For this review, take the finished solid that the model builds, in its own axes (mm). Face numbers are marked on the shaded views. A direction names the side the tool comes from. Coordinates: 2 decimals unless noted, no trailing zeros. Write each loop counter-clockwise with the first axis right and the second up, starting at its lowest first coordinate (ties: lowest second). Pieces come first, ordered by that corner, then holes. Notation, with made-up numbers: M 74.25,3.5 L 126.25,3.5 A20 cw 126.25,33.5 Z; hole C -1,31 d5. An arc over 180 degrees is marked long. One line per question, with ' | ' between items.
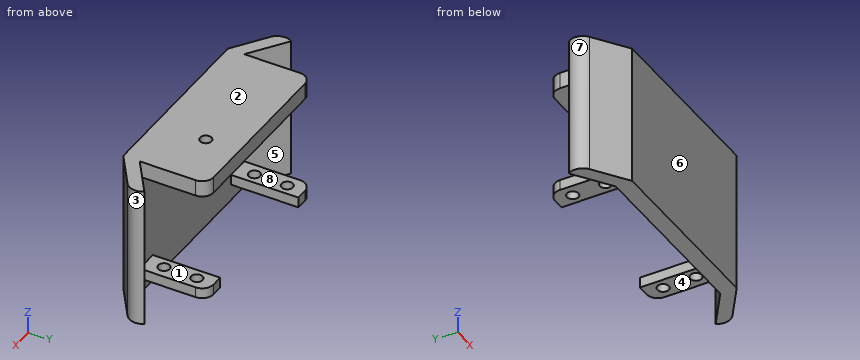
from build123d import *

# Parameters (mm, degrees)
SKETCH1_W            = 55.5
SKETCH1_H            = 43.2
BASE_DEPTH           = 5
SKETCH2_W            = 55.5
SKETCH2_H            = 25.5
WALL_DEPTH           = 5
SKETCH3_W            = 7
SKETCH3_H            = 20.5
MOUNTINGTABS_DEPTH   = 5
LIPS_REACH           = 76.811
SKETCH5_R            = 1.75
MOUNTINGHOLES_DEPTH  = 5
FILLETS_R            = 3.5
SKETCH6_R            = 1.75
THROUGHHOLE_DEPTH    = 5
MIRROR1_START        = -40
MIRROR1_OUTLINE_R    = 1.75
MIRROR1_DEPTH        = 1.8
MIRROR1_START_2      = -38.2
MIRROR1_2_OUTLINE_R  = 1.75
MIRROR1_2_DEPTH      = 3.2
FILLETS_OF_MIRROR2_R = 3.5
CUT_EXTRUDE2_DEPTH   = 5
CUT_EXTRUDE3_DEPTH   = 3.2


# Read off the part's stored shape, not the designer's step: Mirror1
with BuildPart() as part:
    # Sketch1 → base (new body)
    with BuildSketch(Plane(origin=(0, 0, 0), x_dir=(1, 0, 0), z_dir=(0, 1, 0))):
        with Locations((27.75, 21.6)):
            Rectangle(SKETCH1_W, SKETCH1_H)
    extrude(amount=BASE_DEPTH)

    # Sketch2 → wall (add)
    with BuildSketch(Plane(origin=(0, 0, -43.2), x_dir=(-1, 0, 0), z_dir=(0, 0, -1))):
        with Locations((-27.75, 12.75)):
            Rectangle(SKETCH2_W, SKETCH2_H)
    wall = extrude(amount=-WALL_DEPTH)

    # Sketch3 → mountingTabs (add)
    with BuildSketch(Plane.XY.offset(-8.2)):
        with Locations((3.5, 15.25)):
            Rectangle(SKETCH3_W, SKETCH3_H)
        with Locations((52, 15.25)):
            Rectangle(SKETCH3_W, SKETCH3_H)
    extrude(amount=MOUNTINGTABS_DEPTH)

    # lips: up to this face of the body (flat: up to its plane)
    lips_end = Plane(part.part.faces().sort_by_distance((27.75, 12.75, -43.2))[0])
    # Sketch4 → lips (add, up to the picked face)
    with BuildSketch(Plane.XY, mode=Mode.PRIVATE) as lips_sk1:
        with BuildLine():
            Line((0, 0), (-10.208884478, 7.148337868))
            ThreePointArc((-10.208884478, 7.148337868), (-11.894564223, 9.792816133), (-11.218174515, 12.85505036))
            Line((-11.218174515, 12.85505036), (0, 5))
            Line((0, 5), (0, 0))
        make_face()
    lips_tool1 = split(extrude(lips_sk1.sketch, amount=-LIPS_REACH, mode=Mode.PRIVATE), bisect_by=lips_end, keep=Keep.BOTH, mode=Mode.PRIVATE)
    # Sketch4 → lips (add, up to the picked face)
    with BuildSketch(Plane.XY, mode=Mode.PRIVATE) as lips_sk2:
        with BuildLine():
            Line((55.5, 5), (66.718174515, 12.85505036))
            ThreePointArc((66.718174515, 12.85505036), (67.394564223, 9.792816133), (65.708884478, 7.148337868))
            Line((65.708884478, 7.148337868), (55.5, 0))
            Line((55.5, 0), (55.5, 5))
        make_face()
    lips_tool2 = split(extrude(lips_sk2.sketch, amount=-LIPS_REACH, mode=Mode.PRIVATE), bisect_by=lips_end, keep=Keep.BOTH, mode=Mode.PRIVATE)
    add(lips_tool1.solids().sort_by(Axis((-5.839287, 6.590277, 0), (0, 0, -1)))[0])
    add(lips_tool2.solids().sort_by(Axis((61.339287, 6.590277, 0), (0, 0, -1)))[0])

    # Sketch5 → mountingHoles (cut)
    with BuildSketch(Plane.XY.offset(-3.2)):
        with Locations((3.75, 20.25)):
            Circle(SKETCH5_R)
        with Locations(Location((3.75, 10.25, 0), (0, 0, 180))):
            Circle(SKETCH5_R)
        with Locations((51.75, 10.25)):
            Circle(SKETCH5_R)
        with Locations(Location((51.75, 20.25, 0), (0, 0, 180))):
            Circle(SKETCH5_R)
    extrude(amount=-MOUNTINGHOLES_DEPTH, mode=Mode.SUBTRACT)

    # fillets
    fillets_edges = [part.edges().sort_by_distance(p)[0] for p in [
        (0, 25.5, -40.7),
        (55.5, 25.5, -40.7),
        (0, 25.5, -5.7),
        (55.5, 25.5, -5.7),
    ]]
    fillet(fillets_edges, radius=FILLETS_R)

    # Sketch6 → throughHole (cut)
    with BuildSketch(Plane.XY.offset(-38.2)):
        with Locations((38.25, 15.25)):
            Circle(SKETCH6_R)
    throughhole = extrude(amount=-THROUGHHOLE_DEPTH, mode=Mode.SUBTRACT)

    # Mirror1 outline → Mirror1 (cut)
    with BuildSketch(Plane.XY.offset(MIRROR1_START)):
        with Locations((51.75, 10.25)):
            Circle(MIRROR1_OUTLINE_R)
        with Locations((51.75, 20.25)):
            Circle(MIRROR1_OUTLINE_R)
        with Locations((3.75, 20.25)):
            Circle(MIRROR1_OUTLINE_R)
        with Locations((3.75, 10.25)):
            Circle(MIRROR1_OUTLINE_R)
    extrude(amount=MIRROR1_DEPTH, mode=Mode.SUBTRACT)

    # Mirror1 2 outline → Mirror1 2 (add)
    # profile 1 of 2: a face of its own
    with BuildSketch(Plane.XY.offset(MIRROR1_START_2)):
        with BuildLine():
            ThreePointArc((55.5, 22), (54.474873734, 24.474873734), (52, 25.5))
            Line((52, 25.5), (48.5, 25.5))
            Line((48.5, 25.5), (48.5, 5))
            Line((48.5, 5), (55.5, 5))
            Line((55.5, 5), (55.5, 22))
        make_face()
        with Locations((51.75, 10.25)):
            Circle(MIRROR1_2_OUTLINE_R, mode=Mode.SUBTRACT)
        with Locations((51.75, 20.25)):
            Circle(MIRROR1_2_OUTLINE_R, mode=Mode.SUBTRACT)
    # profile 2 of 2: a face of its own
    with BuildSketch(Plane.XY.offset(MIRROR1_START_2)):
        with BuildLine():
            Line((7, 5), (7, 25.5))
            Line((7, 25.5), (3.5, 25.5))
            ThreePointArc((3.5, 25.5), (1.025126266, 24.474873734), (0, 22))
            Line((0, 22), (0, 5))
            Line((0, 5), (7, 5))
        make_face()
        with Locations((3.75, 10.25)):
            Circle(MIRROR1_2_OUTLINE_R, mode=Mode.SUBTRACT)
        with Locations((3.75, 20.25)):
            Circle(MIRROR1_2_OUTLINE_R, mode=Mode.SUBTRACT)
    extrude(amount=MIRROR1_2_DEPTH)

    # Mirror2: wall, throughHole across plane
    add(wall.mirror(Plane(origin=(0, 0, -21.6), x_dir=(1, 0, 0), z_dir=(0, 0, -1))))
    add(throughhole.mirror(Plane(origin=(0, 0, -21.6), x_dir=(1, 0, 0), z_dir=(0, 0, -1))), mode=Mode.SUBTRACT)

    # fillets of Mirror2
    fillets_of_mirror2_edges = [part.edges().sort_by_distance(p)[0] for p in [
        (0, 25.5, -2.5),
        (55.5, 25.5, -2.5),
        (0, 25.5, -37.5),
        (55.5, 25.5, -37.5),
    ]]
    fillet(fillets_of_mirror2_edges, radius=FILLETS_OF_MIRROR2_R)

    # Sketch7 → Cut-Extrude2 (cut)
    with BuildSketch(Plane(origin=(0, 0, -43.2), x_dir=(-1, 0, 0), z_dir=(0, 0, -1))):
        with BuildLine():
            Line((-55.5, 5), (0, 5))
            Line((0, 5), (0, 22))
            ThreePointArc((0, 22), (-1.025126266, 24.474873734), (-3.5, 25.5))
            Line((-3.5, 25.5), (-52, 25.5))
            ThreePointArc((-52, 25.5), (-54.474873734, 24.474873734), (-55.5, 22))
            Line((-55.5, 22), (-55.5, 5))
        make_face()
    extrude(amount=-CUT_EXTRUDE2_DEPTH, mode=Mode.SUBTRACT)

    # Sketch8 → Cut-Extrude3 (cut)
    with BuildSketch(Plane(origin=(0, 0, -8.2), x_dir=(-1, 0, 0), z_dir=(0, 0, -1))):
        with BuildLine():
            Line((-48.5, 25.5), (-52, 25.5))
            ThreePointArc((-52, 25.5), (-54.474873734, 24.474873734), (-55.5, 22))
            Line((-55.5, 22), (-55.5, 5))
            Line((-55.5, 5), (-48.5, 5))
            Line((-48.5, 5), (-48.5, 25.5))
        make_face()
        with BuildLine():
            Line((0, 5), (0, 22))
            ThreePointArc((0, 22), (-1.025126266, 24.474873734), (-3.5, 25.5))
            Line((-3.5, 25.5), (-7, 25.5))
            Line((-7, 25.5), (-7, 5))
            Line((-7, 5), (0, 5))
        make_face()
    extrude(amount=-CUT_EXTRUDE3_DEPTH, mode=Mode.SUBTRACT)


solid = part.part
1. Draft analysis for pull direction X (two halves, no side actions). For the marked faces 6, 7 and 8, state which applies: pulls with the +X half, pulls with the -X half, needs draft (parallel to the pull), parting line crosses it, or undercut.
Computed values:
face 6: needs draft | face 7: pulls with the -X half | face 8: undercut
2. Take a section at A-A on y = 20.25. State the section outline as (x, z) points, plus the area to 3 significant figures.
Computed values:
outline: M 0,-38.2 L 2,-38.2 L 2,-35 L 0,-35 Z; M 0,-5 L 55.5,-5 L 55.5,0 L 0,0 Z; M 5.5,-38.2 L 7,-38.2 L 7,-35 L 5.5,-35 Z; M 48.5,-38.2 L 50,-38.2 L 50,-35 L 48.5,-35 Z; M 53.5,-38.2 L 55.5,-38.2 L 55.5,-35 L 53.5,-35 Z | area: 300 mm2
3. Take a section at C-C on z = -15.5. State the section outline as (x, y) points, plus the area to 3 significant figures.
Computed values:
outline: M -11.22,12.86 A4.1 ccw -10.21,7.15 L 0,0 L 55.5,0 L 65.71,7.15 A4.1 ccw 66.72,12.86 L 55.5,5 L 0,5 Z | area: 394 mm2
4. For line 1 along Y through (x, z) = (3.75, -36.55); line 2 along X through (y, z) = (20.25, -36.8); line 3 along Z through (x, y) = (54, 12), list the stretches that pass through material, from the lowest coordinate up.
Computed values:
line 1: y = 0 to 8.5, 12 to 18.5, 22 to 25.5 | line 2: x = 0 to 2, 5.5 to 7, 48.5 to 50, 53.5 to 55.5 | line 3: z = -38.2 to -35, -5 to 0
5. Clearance check with flat-ended pins moving along their axes: P1, Ø1, axis at x = 15, y = 22.5, coming from the +Z side; P2, Ø19, axis at x = 28, z = -29, coming from the +Y side; P3, Ø5.5, axis at x = 51.75, y = 10.25, coming from the -Z side; P4, Ø6, axis at y = 5.5, z = -25.5, coming from the +X side. State where each tip first meets the part, or that it passes through.
Computed values:
P1: stops at z = 0 | P2: stops at y = 5 | P3: stops at z = -38.2 | P4: stops at x = 66.93
6. Machinability: for the marked faces 1, 2, 3, 4 and 5, which of the approach directions +Z, -Z, +X, -X, +Y, -Y give a long, thin tool a straight path to every point of the face, cutting with its end or side? Answer none if there is none.
Computed values:
face 1: +Y | face 2: +Z, +X, -X, +Y, -Y | face 3: +Z, -Z, +X | face 4: -Z, +Y | face 5: +Z, -Z, +Y
7. Take a section at D-D on y = 15.25. State the section outline as (x, z) points.
Computed values:
outline: M 0,-38.2 L 7,-38.2 L 7,-35 L 0,-35 Z; M 0,-5 L 36.5,-5 L 36.5,0 L 0,0 Z; M 40,-5 L 55.5,-5 L 55.5,0 L 40,0 Z; M 48.5,-38.2 L 55.5,-38.2 L 55.5,-35 L 48.5,-35 Z
8. Take a section at B-B on x = 38.25. State the section outline as (y, z) points, plus the area to 3 significant figures.
Computed values:
outline: M 0,-43.2 L 5,-43.2 L 5,-5 L 13.5,-5 L 13.5,0 L 0,0 Z; M 17,-5 L 25.5,-5 L 25.5,0 L 17,0 Z | area: 301 mm2
